```python
from build123d import *

# Parameters (mm, degrees)
SKETCH_1_W          = 130
SKETCH_1_H          = 60
EXTRUDE_1_DEPTH     = 2
SKETCH_2_R          = 1.65
CUT_EXTRUDE_1_DEPTH = 72.617037079
SKETCH_3_R          = 1.7
CUT_EXTRUDE_2_DEPTH = 72.617037079
SKETCH_4_W          = 31
SKETCH_4_H          = 52
SKETCH_4_W_2        = 28
SKETCH_4_H_2        = 28
CUT_EXTRUDE_4_DEPTH = 72.617037079
EXTRUDE_1_2_DEPTH   = 2
FILLET_1_R          = 1.6
SKETCH_6_W          = 130
SKETCH_6_H          = 2
EXTRUDE_2_DEPTH     = 5


with BuildPart() as part:
    # 草图1 → Extrude 1 (new body)
    with BuildSketch(Plane.XY):
        Rectangle(SKETCH_1_W, SKETCH_1_H)
    extrude(amount=EXTRUDE_1_DEPTH)

    # 草图2 → 切除-拉伸1 (cut, through all)
    with BuildSketch(Plane.XY.offset(2)):
        with Locations((-57, -10)):
            Circle(SKETCH_2_R)
        with Locations((-57, -20)):
            Circle(SKETCH_2_R)
        with Locations(Location((57, -10, 0), (0, 0, 180))):
            Circle(SKETCH_2_R)
        with Locations(Location((57, -20, 0), (0, 0, 180))):
            Circle(SKETCH_2_R)
        with Locations((57, 20)):
            Circle(SKETCH_2_R)
        with Locations((57, 10)):
            Circle(SKETCH_2_R)
        with Locations(Location((-57, 20, 0), (0, 0, 180))):
            Circle(SKETCH_2_R)
        with Locations(Location((-57, 10, 0), (0, 0, 180))):
            Circle(SKETCH_2_R)
    extrude(amount=-CUT_EXTRUDE_1_DEPTH, mode=Mode.SUBTRACT)

    # 草图3 → 切除-拉伸2 (cut, through all)
    with BuildSketch(Plane.XY.offset(2)):
        with Locations((-18, 18)):
            Circle(SKETCH_3_R)
        with Locations((-18, -18)):
            Circle(SKETCH_3_R)
        with Locations((18, 18)):
            Circle(SKETCH_3_R)
        with Locations((18, -18)):
            Circle(SKETCH_3_R)
    extrude(amount=-CUT_EXTRUDE_2_DEPTH, mode=Mode.SUBTRACT)

    # 草图4 → 切除-拉伸4 (cut, through all)
    with BuildSketch(Plane.XY.offset(2)):
        with Locations((-37.5, 0)):
            Rectangle(SKETCH_4_W, SKETCH_4_H)
        with Locations((37.5, 0)):
            Rectangle(SKETCH_4_W, SKETCH_4_H)
        Rectangle(SKETCH_4_W_2, SKETCH_4_H_2)
        Polygon((-15, 26), (-12.5, 18), (12.5, 18), (15, 26), align=None)
        Polygon((12.5, -18), (15, -26), (-15, -26), (-12.5, -18), align=None)
    extrude(amount=-CUT_EXTRUDE_4_DEPTH, mode=Mode.SUBTRACT)

    # 草图5 → Extrude 1 2 (add, through all)
    with BuildSketch(Plane.XY.offset(2)):
        Polygon((-54.717893948, 24.975870915), (-23.717893948, -27.024129085), (-20.282106052, -24.975870915), (-51.282106052, 27.024129085), align=None)
        Polygon((-23.717893948, 27.024129085), (-54.717893948, -24.975870915), (-51.282106052, -27.024129085), (-20.282106052, 24.975870915), align=None)
        Polygon((20.282106052, 24.975870915), (51.282106052, -27.024129085), (54.717893948, -24.975870915), (23.717893948, 27.024129085), align=None)
        Polygon((23.717893948, -27.024129085), (54.717893948, 24.975870915), (51.282106052, 27.024129085), (20.282106052, -24.975870915), align=None)
        Polygon((-15.414213562, 12.585786438), (12.585786438, -15.414213562), (15.414213562, -12.585786438), (-12.585786438, 15.414213562), align=None)
        Polygon((-12.585786438, -15.414213562), (15.414213562, 12.585786438), (12.585786438, 15.414213562), (-15.414213562, -12.585786438), align=None)
    extrude(amount=-EXTRUDE_1_2_DEPTH)

    # 圆角1
    fillet_1_edges = [part.edges().sort_by_distance(p)[0] for p in [
        (-12.5, -18, 1),
        (12.5, -18, 1),
        (15, -26, 1),
        (-15, -26, 1),
        (-15, 26, 1),
        (15, 26, 1),
        (12.5, 18, 1),
        (-12.5, 18, 1),
        (-53, -22.094242357, 1),
        (-53, 22.094242357, 1),
        (-50.671567559, -26, 1),
        (-24.328432441, -26, 1),
        (-22, 22.094242357, 1),
        (-22, -22.094242357, 1),
        (-24.328432441, 26, 1),
        (-50.671567559, 26, 1),
        (-37.5, 3.905757643, 1),
        (-35.171567559, 0, 1),
        (-37.5, -3.905757643, 1),
        (-39.828432441, 0, 1),
        (53, -22.094242357, 1),
        (53, 22.094242357, 1),
        (24.328432441, 26, 1),
        (50.671567559, 26, 1),
        (22, 22.094242357, 1),
        (22, -22.094242357, 1),
        (50.671567559, -26, 1),
        (24.328432441, -26, 1),
        (37.5, -3.905757643, 1),
        (35.171567559, 0, 1),
        (37.5, 3.905757643, 1),
        (39.828432441, 0, 1),
        (11.171572875, 14, 1),
        (-11.171572875, 14, 1),
        (-14, -11.171572875, 1),
        (-14, 11.171572875, 1),
        (-11.171572875, -14, 1),
        (11.171572875, -14, 1),
        (14, 11.171572875, 1),
        (14, -11.171572875, 1),
        (2.828427125, 0, 1),
        (0, -2.828427125, 1),
        (-2.828427125, 0, 1),
        (0, 2.828427125, 1),
    ]]
    fillet(fillet_1_edges, radius=FILLET_1_R)

    # 草图6 → 凸台-拉伸2 (add)
    with BuildSketch(Plane(origin=(0, 30, 0), x_dir=(1, 0, 0), z_dir=(0, 1, 0))):
        with Locations((0, -1)):
            Rectangle(SKETCH_6_W, SKETCH_6_H)
    extrude(amount=EXTRUDE_2_DEPTH)


solid = part.part
```
Geometry check sheet. Reference: the model listing, model coordinates, mm. Round coordinates to 2 decimals unless told otherwise and drop trailing zeros. Loops run counter-clockwise (first coordinate to the right, second up) from the corner with the lowest first, then second, coordinate; pieces in that order, holes last. Notation, with made-up numbers: (48.25, 87.25) - (80.25, 87.25) arc R33 cw to (80.25, 124.25) - close; hole circle Ø7 at (-27, 77). An arc over 180 degrees is marked (long way). Write each question's results on one line, items separated by ' | '. Start each with the question number.
Q1. Thickness scan on line 1 (Y direction, x = 57, z = 0.85); line 2 (Y direction, x = -18, z = 0.8); line 3 (Y direction, x = -32, z = 0.2). Record the ranges inside material, lowest first. Write a range as [from, to].
Q2. Cross-section at C-C on x = -44. Enter the section's corners in (y, z), and give its area (3 significant figures).
Q3. Cross-section at B-B on x = -57. Enter the section's corners in (y, z).
Q4. Release check for a two-part mould opening along X. For faces 1 (the cylindrical face through (-58.65, -19.93, 1.01)), 2 (the flat face through (-1, 2, 0)), 3 (the flat face through (4.73, -7.56, 1.01)) record: +X half, -X half, draft (parallel to the pull), parting line (faces both ways), or undercut.
Q5. Cross-section at D-D on z = 1.55. State how many separate pieces and enclosed holes the cut face has, and give its area (3 significant figures).
Q6. Cross-section at A-A on x = -18. Enter the section's corners in (y, z).
Answers below:
1) line 1: y = [-30, -21.65], [-18.35, -11.65], [-8.35, 8.35], [11.65, 18.35], [21.65, 35] | line 2: y = [-30, -19.7], [-16.3, 16.3], [19.7, 35] | line 3: y = [-30, -26], [-13.13, -5.32], [5.32, 13.13], [26, 35]
2) outline: (-30, 0) - (-26, 0) - (-26, 2) - (-30, 2) - close; (-14.81, 0) - (-7, 0) - (-7, 2) - (-14.81, 2) - close; (7, 0) - (14.81, 0) - (14.81, 2) - (7, 2) - close; (26, 0) - (35, 0) - (35, 2) - (26, 2) - close | area: 57.2 mm²
3) outline: (-30, 0) - (-21.65, 0) - (-21.65, 2) - (-30, 2) - close; (-18.35, 0) - (-11.65, 0) - (-11.65, 2) - (-18.35, 2) - close; (-8.35, 0) - (8.35, 0) - (8.35, 2) - (-8.35, 2) - close; (11.65, 0) - (18.35, 0) - (18.35, 2) - (11.65, 2) - close; (21.65, 0) - (35, 0) - (35, 2) - (21.65, 2) - close
4) face 1: undercut | face 2: draft | face 3: undercut
5) separate pieces: 1 | enclosed holes: 26 | area: 5,180 mm²
6) outline: (-30, 0) - (-19.7, 0) - (-19.7, 2) - (-30, 2) - close; (-16.3, 0) - (16.3, 0) - (16.3, 2) - (-16.3, 2) - close; (19.7, 0) - (35, 0) - (35, 2) - (19.7, 2) - close
